Print and shaded views of the part. All mm, measured from the part's lowest x, y and z. A direction names the side the tool comes from. Coordinates: 2 decimals unless noted, no trailing zeros. Order: outer loops, then holes, each group sorted by start corner. A loop starts at its lowest first (then second) coordinate and runs counter-clockwise, first axis right, second up. Notation, with made-up numbers: M 80.25,54.25 L 124.25,54.25 A25 cw 124.25,82.25 Z; hole C 28.25,30.25 d11. An arc over 180 degrees is marked long. Return JSON: item names as keys, results as strings.
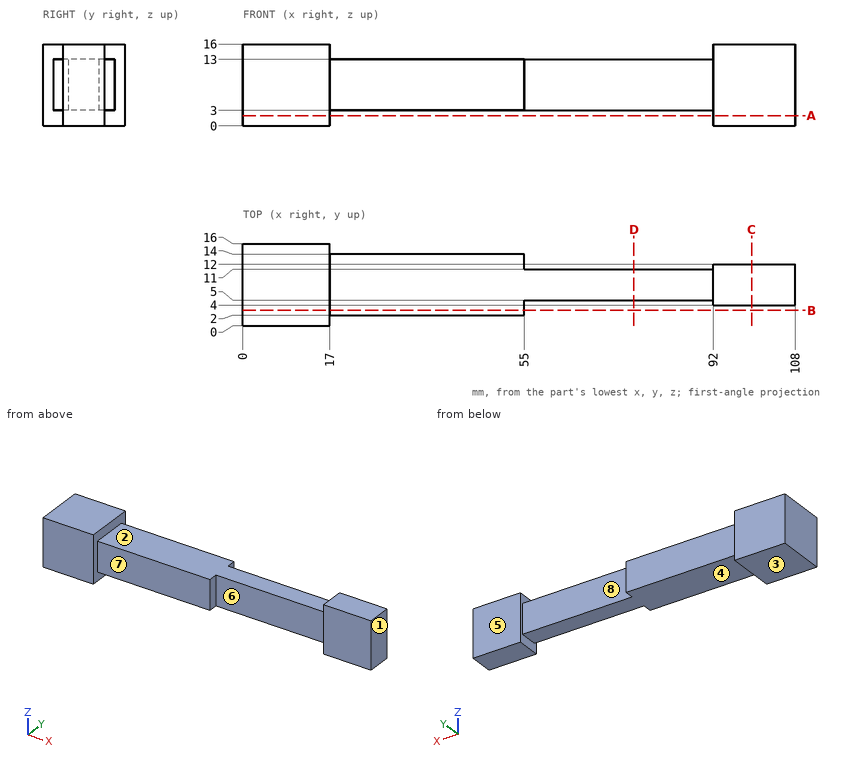
Item 1: Drop flat-ended pins along their axis: pin 1 Ø8 at (x, z) = (97, 5.5) entering from +Y; pin 2 Ø0.9 at (y, z) = (3.5, 6) entering from +X; pin 3 Ø2.5 at (y, z) = (6.5, 11) entering from -X; pin 4 Ø2 at (x, y) = (54.5, 9.5) entering from -Z. Give the stop position or say it passes through.
Check result:
{"pin 1": "stops at y = 12", "pin 2": "stops at x = 55", "pin 3": "stops at x = 0", "pin 4": "stops at z = 3"}
Item 2: Saw through at B-B (y = 3). Write the cut outline in (x, z), and give its area (3 significant figures).
Check result:
{"outline": "M 0,0 L 17,0 L 17,3 L 55,3 L 55,13 L 17,13 L 17,16 L 0,16 Z", "area": "652 mm2"}
Item 3: Saw through at A-A (z = 2). Write the cut outline in (x, y).
Check result:
{"outline": "M 0,0 L 17,0 L 17,16 L 0,16 Z; M 92,4 L 108,4 L 108,12 L 92,12 Z"}
Item 4: Wall check: line 1 (X direction, y = 11.5, z = 2); line 2 (Y direction, x = 57, z = 11.5); line 3 (Z direction, x = 21.5, y = 13.5). Give the ranges that are in metal, low to high.
Check result:
{"line 1": "x = 0 to 17, 92 to 108", "line 2": "y = 5 to 11", "line 3": "z = 3 to 13"}
Item 5: 3-axis set-ups, long thin cutter, end or side, ignore diameter. For the marked faces 4, 5, 6, 7 and 8: which of +Z, -Z, +X, -X, +Y, -Y reach the whole face in a straight line?
Check result:
{"face 4": "-Z, +Y, -Y", "face 5": "+Z, -Z, +X, +Y", "face 6": "+Z, -Z, -Y", "face 7": "+Z, -Z, +X, -Y", "face 8": "+Z, -Z, +Y"}
Item 6: Saw through at C-C (x = 99.5). Write the cut outline in (y, z).
Check result:
{"outline": "M 4,0 L 12,0 L 12,16 L 4,16 Z"}
Item 7: Saw through at D-D (x = 76.5). Write the cut outline in (y, z).
Check result:
{"outline": "M 5,3 L 11,3 L 11,13 L 5,13 Z"}
Item 8: Pull direction X, two halves, no side cores. Call the marked faces 1, 2 and 3: +X half, -X half, draft (parallel to the pull), parting line (faces both ways), or undercut.
Check result:
{"face 1": "+X half", "face 2": "undercut", "face 3": "draft"}
